```python
from build123d import *

# Parameters (mm, degrees)
F0_R      = 96.551429
F1_DEPTH  = 60.706
F4_DEPTH  = 16.764
F5_DEPTH  = 18.288
F7_DEPTH  = 29.718
F9_DEPTH  = 24.892
F10_DEPTH = 25.4


with BuildPart() as f1:
    # F0 (on Top) → F1 (new body)
    with BuildSketch(Plane.XY):
        Circle(F0_R)
    extrude(amount=-F1_DEPTH)

    # F3 (on face) → F4 (cut)
    with BuildSketch(Plane.XY):
        with BuildLine():
            Line((0, -72.571998), (0, -82.988975))
            ThreePointArc((0, -82.988975), (11.31764, -80.094339), (20.304218, -72.630472))
            Line((20.304218, -72.630472), (0, -72.571998))
        make_face()
    extrude(amount=-F4_DEPTH, mode=Mode.SUBTRACT)

    # F3 (on face) → F5 (cut)
    with BuildSketch(Plane.XY):
        with BuildLine():
            Line((20.304218, -72.630472), (-21.942582, -72.508805))
            ThreePointArc((-21.942582, -72.508805), (-0.849221, -83.000085), (20.304218, -72.630472))
        make_face()
    extrude(amount=-F5_DEPTH, mode=Mode.SUBTRACT)

    # F6 (on Top) → F7 (cut)
    with BuildSketch(Plane.XY):
        with BuildLine():
            Line((-23.170974, 76.51294), (18.255305, 76.043338))
            ThreePointArc((18.255305, 76.043338), (-2.257895, 93.915969), (-23.170974, 76.51294))
        make_face()
    extrude(amount=-F7_DEPTH, mode=Mode.SUBTRACT)

    # F8 (on Top) → F9 (cut)
    with BuildSketch(Plane.XY):
        with BuildLine():
            Line((64.235799, 20.705102), (66.905841, -17.182859))
            ThreePointArc((66.905841, -17.182859), (75.55273, 2.464567), (64.235799, 20.705102))
        make_face()
        with BuildLine():
            ThreePointArc((-64.235799, 20.705102), (-75.55273, 2.464567), (-66.905841, -17.182859))
            Line((-66.905841, -17.182859), (-64.235799, 20.705102))
        make_face()
    extrude(amount=-F9_DEPTH, mode=Mode.SUBTRACT)

    # F8 (on Top) → F10 (cut)
    with BuildSketch(Plane.XY):
        with BuildLine():
            Line((64.235799, 20.705102), (66.905841, -17.182859))
            ThreePointArc((66.905841, -17.182859), (75.55273, 2.464567), (64.235799, 20.705102))
        make_face()
        with BuildLine():
            ThreePointArc((-64.235799, 20.705102), (-75.55273, 2.464567), (-66.905841, -17.182859))
            Line((-66.905841, -17.182859), (-64.235799, 20.705102))
        make_face()
    extrude(amount=-F10_DEPTH, mode=Mode.SUBTRACT)


solid = f1.part
```
Part model, mm, in its own coordinate system. A direction names the side the tool comes from. Round coordinates to 2 decimals unless told otherwise and drop trailing zeros. Loops run counter-clockwise (first coordinate to the right, second up) from the corner with the lowest first, then second, coordinate; pieces in that order, holes last. Notation, with made-up numbers: (-1, 82.5) -> (47, 82.5) arc R26 cw to (47, 120.5) -> close; hole circle Ø9 at (17, 74.25). An arc over 180 degrees is marked (long way). Use CSV: the item, a comma, the result in double quotes. Start each with the question number.
1) Cut at C-C, the plane y = 0. Write the cut outline in (x, z).
2) Cut at D-D, the plane x = 31.5. Write the cut outline in (y, z), plus the area to 3 significant figures.
3) Pull direction Y, two halves, no side cores. Call faces 1 (the cylindrical face through (75.573, 2.153, -12.522)), 2 (the flat face through (-1, 1, -60.706)), 3 (the cylindrical face through (92.093, 29.001, -29.928)): +Y half, -Y half, draft (parallel to the pull), parting line (faces both ways), or undercut.
4) Wall check: L1, parallel to Y at x = -8.5, z = -15; L2, parallel to X at y = 1.5, z = -31; L3, parallel to Y at x = -1, z = -48. Give the ranges that are in metal, low to high. Write a range as [from, to].
5) Cut at A-A, the plane z = -11.5. Write the cut outline in (x, y), plus the area to 3 significant figures.
6) Drop flat-ended pins along their axis: P1, Ø10, axis at x = -28, z = -42, coming from the -Y side; P2, Ø8, axis at x = -40.5, z = -6, coming from the -Y side; P3, Ø5.5, axis at x = 70.5, y = -3.5, coming from the +Z side. Give the stop position or say it passes through.
7) Cut at B-B, the plane z = -22.5. Write the cut outline in (x, y).
8) Which spindle directions (+Z, -Z, +X, -X, +Y, -Y) get a long thin tool onto all of the face, cutting with end or side? Do faces 4 (the flat face through (-1, 1, 0)), 5 (the flat face through (-1, -77, -18.288)). Say none if no direction does.
Determined:
1,outline,"(-96.55, -60.71) -> (96.55, -60.71) -> (96.55, 0) -> (75.59, 0) -> (75.59, -25.4) -> (65.69, -25.4) -> (65.69, 0) -> (-65.69, 0) -> (-65.69, -25.4) -> (-75.59, -25.4) -> (-75.59, 0) -> (-96.55, 0) -> close"
2,outline,"(-91.27, -60.71) -> (91.27, -60.71) -> (91.27, 0) -> (-91.27, 0) -> close"
2,area,"11,100 mm2"
3,face 1,"undercut"
3,face 2,"draft"
3,face 3,"parting line"
4,L1,"y = [-96.18, -81.85], [-72.55, 76.35], [93.04, 96.18]"
4,L2,"x = [-96.54, 96.54]"
4,L3,"y = [-96.55, 96.55]"
5,outline,"circle Ø193.1 at (0, 0); hole (-66.91, -17.18) -> (-64.24, 20.71) arc R23.02 ccw to start; hole (-23.17, 76.51) -> (18.26, 76.04) arc R20.98 ccw to start; hole (-21.94, -72.51) arc R26.6 ccw to (0, -82.99) arc R26.6 ccw to (20.3, -72.63) -> close; hole (64.24, 20.71) -> (66.91, -17.18) arc R23.02 ccw to start"
5,area,"27,900 mm2"
6,P1,"stops at y = -93.77"
6,P2,"stops at y = -89.39"
6,P3,"stops at z = -25.4"
7,outline,"circle Ø193.1 at (0, 0); hole (-66.91, -17.18) -> (-64.24, 20.71) arc R23.02 ccw to start; hole (-23.17, 76.51) -> (18.26, 76.04) arc R20.98 ccw to start; hole (64.24, 20.71) -> (66.91, -17.18) arc R23.02 ccw to start"
8,face 4,"+Z, +X, -X, +Y, -Y"
8,face 5,"+Z"
